Can you work these out from the model? Positions are in its coordinate system, mm. A direction names the side the tool comes from. Round coordinates to 2 decimals unless told otherwise and drop trailing zeros. Loops run counter-clockwise (first coordinate to the right, second up) from the corner with the lowest first, then second, coordinate; pieces in that order, holes last. Notation, with made-up numbers: (74, 65.25) -> (129, 65.25) arc R25 cw to (129, 79.25) -> close; hole circle Ø1 at (-10.5, 10). An arc over 180 degrees is marked (long way). Use a Markdown table: item, result.
from build123d import *

# Parameters (mm, degrees)
SKETCH1_R           = 4
SKETCH1_R_2         = 0.8
BOSS_EXTRUDE1_DEPTH = 6.4
BOSS_EXTRUDE2_DEPTH = 1.6
CIRPATTERN1_COUNT   = 6
SKETCH3_R           = 23.654175107
SKETCH3_R_2         = 22
CUT_EXTRUDE1_DEPTH  = 6.4


with BuildPart() as part:
    # Sketch1 → Boss-Extrude1 (new body)
    with BuildSketch(Plane(origin=(0, 0, 0), x_dir=(1, 0, 0), z_dir=(0, 1, 0))):
        Circle(SKETCH1_R)
        Circle(SKETCH1_R_2, mode=Mode.SUBTRACT)
    extrude(amount=BOSS_EXTRUDE1_DEPTH)

    # Sketch2 → Boss-Extrude2 (add, symmetric)
    with BuildSketch(Plane.XY):
        Polygon((-4, 0), (-23.6, 19.6), (-23.6, 21.2), (-22, 21.2), (-22, 27.6), (-18.8, 27.6), (-18.8, 24.4), (-0.8, 6.4), (-0.8, 0), align=None)
    boss_extrude2 = extrude(amount=BOSS_EXTRUDE2_DEPTH, both=True)

    # CirPattern1: Boss-Extrude2 ×6 about axis
    cirpattern1_axis = Axis((0, 0, 0), (0, 1, 0))
    for i in range(1, CIRPATTERN1_COUNT):
        add(boss_extrude2.rotate(cirpattern1_axis, i * 360 / CIRPATTERN1_COUNT))

    # Sketch3 → Cut-Extrude1 (cut)
    with BuildSketch(Plane(origin=(0, 27.6, 0), x_dir=(1, 0, 0), z_dir=(0, 1, 0))):
        Circle(SKETCH3_R)
        Circle(SKETCH3_R_2, mode=Mode.SUBTRACT)
    extrude(amount=-CUT_EXTRUDE1_DEPTH, mode=Mode.SUBTRACT)


solid = part.part
1. Which directions (+Z, -Z, +X, -X, +Y, -Y) give clear straight access to the entire face, cutting with the end or side of a thin tool? Please do faces 1 (the flat face through (-9.9, 15.5, 0)), 2 (the flat face through (11, 21.2, 20)), 3 (the flat face through (11.78, 20.39, -20.45)).
Answer sheet:
| item | result |
|---|---|
| face 1 | +Y |
| face 2 | +Z, +X, +Y |
| face 3 | -Z, +X, +Y, -Y |
2. I want a section at B-B (y = 3). Please give me the cut outline in (x, z), plus the area to 3 significant figures.
Answer sheet:
| item | result |
|---|---|
| outline | (-7, -1.6) -> (-3.67, -1.6) arc R4 ccw to (-3.22, -2.37) -> (-4.89, -5.26) -> (-2.11, -6.86) -> (-0.45, -3.97) arc R4 ccw to (0.45, -3.97) -> (2.11, -6.86) -> (4.89, -5.26) -> (3.22, -2.37) arc R4 ccw to (3.67, -1.6) -> (7, -1.6) -> (7, 1.6) -> (3.67, 1.6) arc R4 ccw to (3.22, 2.37) -> (4.89, 5.26) -> (2.11, 6.86) -> (0.45, 3.97) arc R4 ccw to (-0.45, 3.97) -> (-2.11, 6.86) -> (-4.89, 5.26) -> (-3.22, 2.37) arc R4 ccw to (-3.67, 1.6) -> (-7, 1.6) -> close; hole circle Ø1.6 at (0, 0) |
| area | 108 mm² |
3. I want a section at C-C (z = 10). Please give me the cut outline in (x, y), plus the area to 3 significant figures.
Answer sheet:
| item | result |
|---|---|
| outline | (-7.62, 8.47) -> (-3.93, 6.62) -> (-3.93, 16.22) -> (-7.62, 18.07) -> close; (3.93, 6.62) -> (7.62, 8.47) -> (7.62, 18.07) -> (3.93, 16.22) -> close |
| area | 70.9 mm² |
4. I want a section at A-A (y = 22). Please give me the cut outline in (x, z), plus the area to 3 significant figures.
Answer sheet:
| item | result |
|---|---|
| outline | (-21.94, -1.6) -> (-16.4, -1.6) -> (-16.4, 1.6) -> (-21.94, 1.6) arc R22 ccw to start; (-12.36, -18.2) arc R22 ccw to (-9.59, -19.8) -> (-6.81, -15) -> (-9.59, -13.4) -> close; (-12.36, 18.2) -> (-9.59, 13.4) -> (-6.81, 15) -> (-9.59, 19.8) arc R22 ccw to start; (6.81, -15) -> (9.59, -19.8) arc R22 ccw to (12.36, -18.2) -> (9.59, -13.4) -> close; (6.81, 15) -> (9.59, 13.4) -> (12.36, 18.2) arc R22 ccw to (9.59, 19.8) -> close; (16.4, -1.6) -> (21.94, -1.6) arc R22 ccw to (21.94, 1.6) -> (16.4, 1.6) -> close |
| area | 107 mm² |
5. If we mould it in two halves opening along Z, with no side actions, what happens to faces 4 (the flat face through (-11, 21.2, -20)), 5 (the cylindrical face through (10.981, 24.445, 19.064)), 6 (the cylindrical face through (-0.63, 3.16, 0.49)), 7 (the flat face through (12, 14, -1.6))? For each: +Z half, -Z half, draft (parallel to the pull), parting line (faces both ways), or undercut.
Answer sheet:
| item | result |
|---|---|
| face 4 | draft |
| face 5 | +Z half |
| face 6 | undercut |
| face 7 | undercut |
6. I need wall thicknesses on line 1 (X direction, y = 4, z = 0); line 2 (Z direction, x = -7, y = 8.75); line 3 (Z direction, x = 20, y = 24). Which ranges of each line are inside material? Lowest first, please.
Answer sheet:
| item | result |
|---|---|
| line 1 | x = -8 to -0.8, 0.8 to 8 |
| line 2 | z = -10.68 to -8.92, -1.6 to 1.6, 8.92 to 10.68 |
| line 3 | z = -1.6 to 1.6 |
7. Will these pins go through, and if not, where does the flat tip stop? pin 1 Ø6 at (x, y) = (17.5, 19) entering from -Z; pin 2 Ø0.6 at (x, z) = (0, -3.5) entering from +Y; pin 3 Ø8 at (x, y) = (1.5, 15.5) entering from +Z.
Answer sheet:
| item | result |
|---|---|
| pin 1 | stops at z = -1.6 |
| pin 2 | stops at y = 8.89 |
| pin 3 | stops at z = 12.73 |
8. I want a section at D-D (x = -15). Please give me the cut outline in (y, z), plus the area to 3 significant figures.
Answer sheet:
| item | result |
|---|---|
| outline | (11, -1.6) -> (20.6, -1.6) -> (20.6, 1.6) -> (11, 1.6) -> close |
| area | 30.7 mm² |
